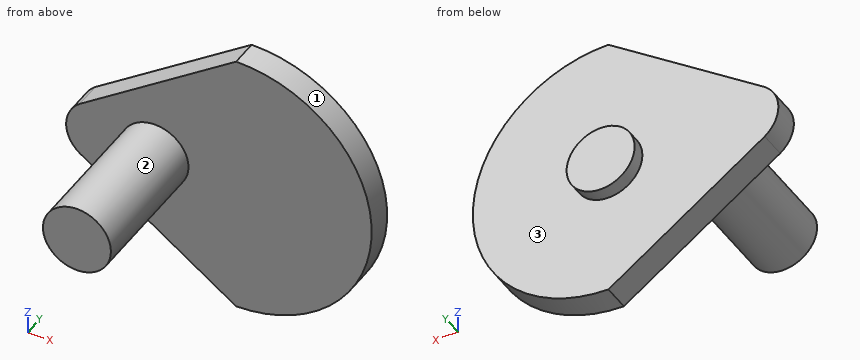
```python
from build123d import *

# Parameters (mm, degrees)
F1_R     = 3.175
F2_DEPTH = 12.7
F4_DEPTH = 2.54
F5_R     = 3.175
F6_DEPTH = 1.27


with BuildPart() as f2:
    # F1 (on Front) → F2 (new body)
    with BuildSketch(Plane.XZ):
        with Locations((-7.62, 0)):
            Circle(F1_R)
    extrude(amount=F2_DEPTH)

    # F3 (on Front) → F4 (join)
    with BuildSketch(Plane.XZ):
        with BuildLine():
            Line((-14.5955, -2.559695), (0, -12.660234))
            ThreePointArc((0, -12.660234), (12.660234, 0), (0, 12.660234))
            Line((0, 12.660234), (-14.5955, 2.559695))
            ThreePointArc((-14.5955, 2.559695), (-15.87429, 0), (-14.5955, -2.559695))
        make_face()
    extrude(amount=-F4_DEPTH)

    # F5 (on face) → F6 (join)
    with BuildSketch(Plane(origin=(0, 2.54, 0), x_dir=(-1, 0, 0), z_dir=(0, 1, 0))):
        Circle(F5_R)
    extrude(amount=F6_DEPTH)


solid = f2.part
```
CAD build for the part. Positions are in the model's coordinates, mm. Face numbers are marked on the shaded views. A direction names the side the tool comes from. Coordinates: 2 decimals unless noted, no trailing zeros. Order: outer loops, then holes, each group sorted by start corner. A loop starts at its lowest first (then second) coordinate and runs counter-clockwise, first axis right, second up. Notation, with made-up numbers: (37.25, 77.25) - (44.25, 77.25) arc R25 cw to (44.25, 113.25) - close; hole circle Ø11 at (46.5, 41). An arc over 180 degrees is marked (long way). Use a Markdown table: item, result. Add a question column.
(1) Flat gauge pins, fed straight in: pin 1 (3 mm diameter, centred on x = -7, z = 6, fed in from +Y); pin 2 (1 mm diameter, centred on y = -8.5, z = -4, fed in from +X); pin 3 (5 mm diameter, centred on y = -7, z = -3.5, fed in from -X); pin 4 (7.5 mm diameter, centred on x = -1.5, z = -3.5, fed in from -Y). Where does each tip first touch, or does it go through?
(2) Saw through at B-B (x = -5.75). Give the cut face in (y, z).
(3) Saw through at A-A (z = 0). Give the cut face in (x, y) (3 decimals), then the cut area to 3 significant figures.
(4) Saw through at C-C (y = -10.5). Give the cut face in (x, z) (3 decimals).
(5) Drill centre lines: line 1 along Y through (x, z) = (-9.25, -2.5); line 2 along Y through (x, z) = (-6.5, -4); line 3 along Z through (x, y) = (-8.5, -1). Where is each one in solid material? Low to high. Write a range as [from, to].
(6) Saw through at D-D (x = -1). Give the cut face in (y, z).
(7) Which spindle directions (+Z, -Z, +X, -X, +Y, -Y) get a long thin tool onto all of the face, cutting with end or side? Do the marked faces 1, 2 and 3. Say none if no direction does.
Solved:
| question | item | result |
|---|---|---|
| 1 | pin 1 | stops at y = 2.54 |
| 1 | pin 2 | passes through |
| 1 | pin 3 | stops at x = -10.63 |
| 1 | pin 4 | stops at y = 0 |
| 2 | outline | (-12.7, -2.57) - (0, -2.57) - (0, -8.68) - (2.54, -8.68) - (2.54, 8.68) - (0, 8.68) - (0, 2.57) - (-12.7, 2.57) - close |
| 3 | outline | (-15.874, 0) - (-10.795, 0) - (-10.795, -12.7) - (-4.445, -12.7) - (-4.445, 0) - (12.66, 0) - (12.66, 2.54) - (3.175, 2.54) - (3.175, 3.81) - (-3.175, 3.81) - (-3.175, 2.54) - (-15.874, 2.54) - close |
| 3 | area | 161 mm² |
| 4 | outline | circle Ø6.35 at (-7.62, 0) |
| 5 | line 1 | y = [-12.7, 2.54] |
| 5 | line 2 | y = [0, 2.54] |
| 5 | line 3 | z = [-3.05, 3.05] |
| 6 | outline | (0, -11.97) - (2.54, -11.97) - (2.54, -3.01) - (3.81, -3.01) - (3.81, 3.01) - (2.54, 3.01) - (2.54, 11.97) - (0, 11.97) - close |
| 7 | face 1 | +X, +Y, -Y |
| 7 | face 2 | -Y |
| 7 | face 3 | +Y |
